Here's how the part is built. I have some questions about the finished solid (model axes, mm). Coordinates: 2 decimals unless noted, no trailing zeros. Write each loop counter-clockwise with the first axis right and the second up, starting at its lowest first coordinate (ties: lowest second). Pieces come first, ordered by that corner, then holes.
Item 1: I want a section at A-A (y = 114.3). Please give me the cut outline in (x, z) (3 decimals), and give its area (3 significant figures).
Item 2: I'm going to push flat-ended pins straight in: P1, Ø1, axis at x = 1.5, y = 155, coming from the -Z side; P2, Ø5.5, axis at y = 114.3, z = -44.45, coming from the +X side; P3, Ø5, axis at x = 6, z = -198, coming from the +Y side; P4, Ø1, axis at x = 4.5, z = -213, coming from the +Y side. Where does each tip first touch, or does it pass through?
Item 3: I want a section at B-B (z = -114.3). Please give me the cut outline in (x, y) (3 decimals), and give its area (3 significant figures).
Item 4: I want a section at D-D (z = -44.45). Please give me the cut outline in (x, y) (3 decimals), and give its area (3 significant figures).
Item 5: I want a section at C-C (y = 44.45). Please give me the cut outline in (x, z) (3 decimals).
Item 6: Please list where these lines run through material, in increasing order: line 1 (Z direction, x = 1.25, y = 42.5); line 2 (Y direction, x = 3.75, z = -44.45) (3 decimals); line 3 (Y direction, x = 4, z = -114.3) (3 decimals).
Item 7: If we mould it in two halves opening along Y, with no side actions, what happens to faces 1 (the face through (6, 125, 0)), 2 (the face through (6.04, 111.2, -43.76)), 3 (the face through (6, 0, -129)), 4 (the face through (6.036, 47.127, -116.007))? For each: pulls with the +Y half, pulls with the -Y half, needs draft (parallel to the pull), parting line crosses it, or undercut.
from build123d import *

# Parameters (mm, degrees)
BOSS_EXTRUDE1_DEPTH         = 11.90625
F_1_4_0_25_DIAMETER_HOLE1_D = 6.35


with BuildPart() as part:
    # Sketch1 → Boss-Extrude1 (new body)
    with BuildSketch(Plane(origin=(0, 0, 0), x_dir=(0, 0, -1), z_dir=(1, 0, 0))):
        Polygon((0, 0), (0, 254), (254, 0), align=None)
    extrude(amount=BOSS_EXTRUDE1_DEPTH)

    # 1/4 (0.25) Diameter Hole1 (through all)
    with Locations(Plane.ZY):
        with Locations((-114.3, 44.45), (-44.45, 114.3), (-44.45, 177.8), (-177.8, 44.45)):
            Hole(F_1_4_0_25_DIAMETER_HOLE1_D / 2)


solid = part.part
Answer:
1. outline: (0, -139.7) - (11.906, -139.7) - (11.906, -47.625) - (0, -47.625) - close; (0, -41.275) - (11.906, -41.275) - (11.906, 0) - (0, 0) - close
1. area: 1,590 mm2
2. P1: stops at z = -99.5
2. P2: passes through
2. P3: stops at y = 58.5
2. P4: stops at y = 41.5
3. outline: (0, 0) - (11.906, 0) - (11.906, 41.275) - (0, 41.275) - close; (0, 47.625) - (11.906, 47.625) - (11.906, 139.7) - (0, 139.7) - close
3. area: 1,590 mm2
4. outline: (0, 0) - (11.906, 0) - (11.906, 111.125) - (0, 111.125) - close; (0, 117.475) - (11.906, 117.475) - (11.906, 174.625) - (0, 174.625) - close; (0, 180.975) - (11.906, 180.975) - (11.906, 209.55) - (0, 209.55) - close
4. area: 2,340 mm2
5. outline: (0, -209.55) - (11.906, -209.55) - (11.906, -180.975) - (0, -180.975) - close; (0, -174.625) - (11.906, -174.625) - (11.906, -117.475) - (0, -117.475) - close; (0, -111.125) - (11.906, -111.125) - (11.906, 0) - (0, 0) - close
6. line 1: z = -211.5 to -180.31, -175.29 to -116.81, -111.79 to 0
6. line 2: y = 0 to 111.125, 117.475 to 174.625, 180.975 to 209.55
6. line 3: y = 0 to 41.275, 47.625 to 139.7
7. face 1: needs draft
7. face 2: undercut
7. face 3: pulls with the -Y half
7. face 4: undercut
